For this review, take the finished solid that the model builds, in its own axes (mm). A direction names the side the tool comes from. Give positions to 0.01 mm unless a question says otherwise; leave off trailing zeros. Order: outer loops, then holes, each group sorted by start corner. A loop starts at its lowest first (then second) coordinate and runs counter-clockwise, first axis right, second up. Notation, with made-up numbers: (-15.75, -27) - (19.25, -27) arc R21 cw to (19.25, -22) - close; hole circle Ø3 at (-18.5, 42). An arc over 180 degrees is marked (long way). One line per item, written item: value.
```python
from build123d import *

# Parameters (mm, degrees)
F1_DEPTH = 25.4
F2_R     = 2.2225
F3_DEPTH = 33.353518
F4_R     = 5.08
F6_R     = 3.81
F7_DEPTH = 43.18
F8_R     = 88.709103
F8_R_2   = 79.375
F9_DEPTH = 25.4


with BuildPart() as f1:
    # F0 (on Front) → F1 (new body)
    with BuildSketch(Plane.XZ):
        Polygon((-63.5, 50.8), (-81.989688, 0), (-56.589688, 0), (-45.033633, 31.75), (45.033633, 31.75), (56.589688, 0), (81.989688, 0), (63.5, 50.8), align=None)
    extrude(amount=F1_DEPTH)

    # F2 (on face) → F3 (cut, through all)
    with BuildSketch(Plane(origin=(0, 0, 0), x_dir=(1, 0, 0), z_dir=(0, 0, -1))):
        with Locations((69.85, 12.7)):
            Circle(F2_R)
        with Locations((-69.85, 12.7)):
            Circle(F2_R)
    extrude(amount=-F3_DEPTH, mode=Mode.SUBTRACT)

    # F4
    f4_edges = [f1.edges().sort_by_distance(p)[0] for p in [
        (-72.744844, -25.4, 25.4),
        (-50.81166, -25.4, 15.875),
        (0, -25.4, 31.75),
        (50.81166, -25.4, 15.875),
        (72.744844, -25.4, 25.4),
        (0, -25.4, 50.8),
        (72.744844, 0, 25.4),
        (50.81166, 0, 15.875),
        (0, 0, 31.75),
        (-50.81166, 0, 15.875),
        (-72.744844, 0, 25.4),
        (0, 0, 50.8),
        (-63.5, -12.7, 50.8),
        (63.5, -12.7, 50.8),
    ]]
    fillet(f4_edges, radius=F4_R)

    # F6 (on offset) → F7 (cut, through all)
    with BuildSketch(Plane.XY.offset(7.62)):
        with Locations((-69.85, -12.7)):
            Circle(F6_R)
        with Locations((69.85, -12.7)):
            Circle(F6_R)
    extrude(amount=F7_DEPTH, mode=Mode.SUBTRACT)

    # F8 (on Top) → F9 (cut)
    with BuildSketch(Plane.XY):
        with Locations((0, -12.65686)):
            Circle(F8_R)
        with Locations((0, -12.65686)):
            Circle(F8_R_2, mode=Mode.SUBTRACT)
    extrude(amount=F9_DEPTH, mode=Mode.SUBTRACT)


solid = f1.part
```
(1) Take a section at C-C (y = -18.5). Write out the cut boundary in (x, z).
Answers below:
outline: (-79.16, 0) - (-56.59, 0) - (-45.03, 31.75) - (45.03, 31.75) - (56.59, 0) - (79.16, 0) - (79.16, 7.78) - (64.72, 47.46) arc R5.08 ccw to (59.94, 50.8) - (-59.94, 50.8) arc R5.08 ccw to (-64.72, 47.46) - (-79.16, 7.78) - close
(2) Draft analysis for pull direction X (two halves, no side actions). For faces 1 (the face through (-73.57, -10.9, 23.13)), 2 (the face through (-1, -13, 31.75)), 3 (the face through (1, -13, 50.8)), state which applies: pulls with the +X half, pulls with the -X half, needs draft (parallel to the pull), parting line crosses it, or undercut.
Answers below:
face 1: pulls with the -X half
face 2: undercut
face 3: needs draft
(3) Take a section at A-A (z = 5.5). Give the number of separate pieces and of enclosed holes in the cut face, then the cut area to 3 significant figures.
Answers below:
separate pieces: 2
enclosed holes: 2
area: 1,180 mm^2
(4) Take a section at B-B (x = -24.5). Write out the cut boundary in (y, z).
Answers below:
outline: (-25.4, 36.83) arc R5.08 ccw to (-20.32, 31.75) - (-5.08, 31.75) arc R5.08 ccw to (0, 36.83) - (0, 45.72) arc R5.08 ccw to (-5.08, 50.8) - (-20.32, 50.8) arc R5.08 ccw to (-25.4, 45.72) - close
(5) Machinability: for faces 4 (the face through (0.68, -23.951, 33.278)), 5 (the face through (-69.9, -15.2, 7.62)), 6 (the face through (50.73, -12.59, 16.1)), 7 (the face through (-72.07, -12.8, 3.76)), which of the approach directions +Z, -Z, +X, -X, +Y, -Y give a long, thin tool a straight path to every point of the face, cutting with its end or side? Answer none if there is none.
Answers below:
face 4: -Z, -Y
face 5: +Z
face 6: -Z, +Y, -Y
face 7: +Z, -Z
(6) For P1, Ø3.5, axis at x = 69.85, y = -12.7, coming from the +Z side; P2, Ø3, axis at y = -6, z = 34, coming from the -X side; P3, Ø12, axis at x = -69.85, y = -12.7, coming from the +Z side; P4, Ø7.5, axis at x = -9.5, y = -10, coming from the -Z side, all flat-tipped, find the tip position at first contact; note any pin that passes through.
Answers below:
P1: passes through
P2: stops at x = -70.16
P3: stops at z = 48.97
P4: stops at z = 31.75
(7) Wall thickness on line 1 (Y direction, x = -69.85, z = 3.75); line 2 (X direction, y = -13.5, z = 7); line 3 (Y direction, x = 69.85, z = 19.5): over which ranges is each line inside the solid? List them lowest first. Write a range as from..to.
Answers below:
line 1: y = -25.4..-14.92, -10.48..0
line 2: x = -79.37..-71.92, -67.78..-54.04, 54.04..67.78, 71.92..79.37
line 3: y = -25.39..-16.51, -8.89..-0.01
